Input: dimensioned drawing with shaded views. Units: mm. Origin: part minimum x, y, z. Round coordinates to 2 decimals unless told otherwise and drop trailing zeros. Order: outer loops, then holes, each group sorted by start corner. A loop starts at its lowest first (then second) coordinate and runs counter-clockwise, first axis right, second up. Notation, with made-up numbers: (85.25, -14.75) - (94.25, -14.75) arc R33 ccw to (94.25, 13.25) - close; hole circle Ø1 at (1, 44.25). An arc over 180 degrees is marked (long way). Put each result on its own line as item: value. Start each with the question number.
(1) Section D-D (x = 16.25). Output: boundary loops of the cut face in (y, z), and give its area (3 significant figures).
(2) Pin query (flat end, axial travel): P1, Ø1.5, axis at x = 5.5, z = 1, coming from the +Y side; P2, Ø1.6, axis at x = 4.5, y = 13.5, coming from the +Z side; P3, Ø1, axis at y = 14, z = 3.5, coming from the -X side; P4, Ø1.5, axis at x = 15, z = 1.5, coming from the +Y side. Return the tip coordinate at first contact, or that it passes through.
(3) Pull-direction query (X, two-part tool) for the marked faces 1, 2 and 3; classes: released by +X, released by -X, zero draft, split by the parting line, or undercut.
(4) Section B-B (x = 4.5). Output: boundary loops of the cut face in (y, z).
(5) Section A-A (z = 3.45). Output: boundary loops of the cut face in (x, y), and give its area (3 significant figures).
(6) Material intervals for L1, parallel to X at y = 4.5, z = 1.4; L2, parallel to Y at x = 4, z = 0.85, sorted ascending. Write a range as [from, to].
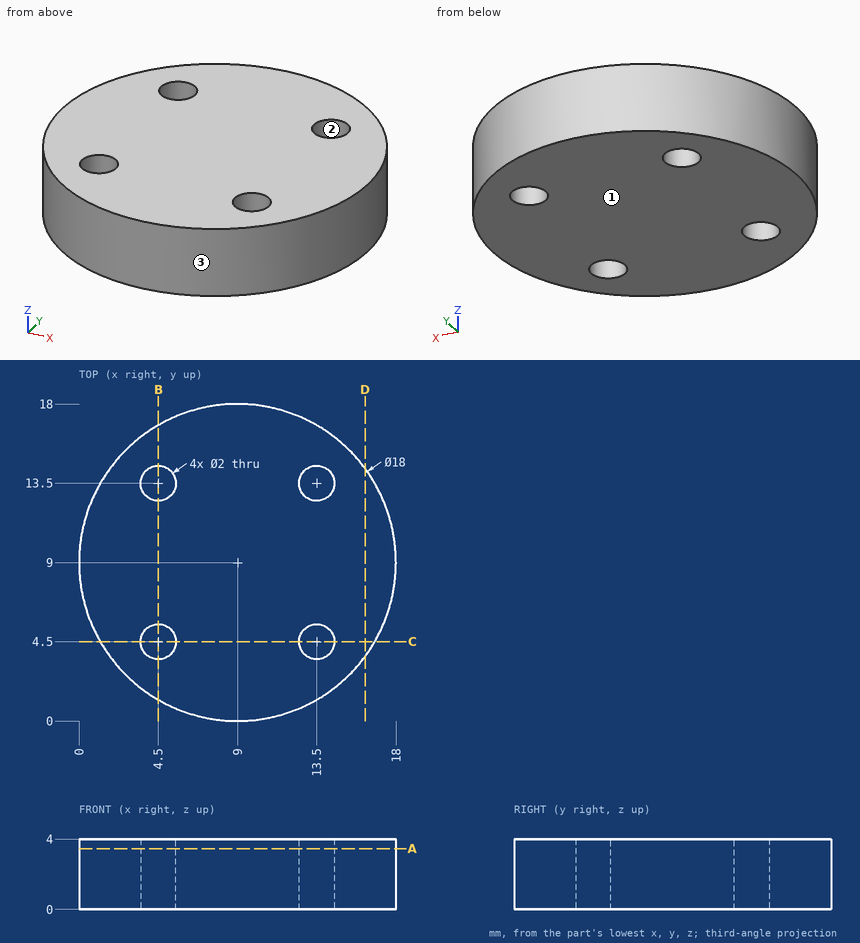
Checks:
1. outline: (3.67, 0) - (14.33, 0) - (14.33, 4) - (3.67, 4) - close
1. area: 42.7 mm²
2. P1: stops at y = 17.57
2. P2: passes through
2. P3: stops at x = 1.21
2. P4: stops at y = 16.31
3. face 1: zero draft
3. face 2: undercut
3. face 3: split by the parting line
4. outline: (1.21, 0) - (3.5, 0) - (3.5, 4) - (1.21, 4) - close; (5.5, 0) - (12.5, 0) - (12.5, 4) - (5.5, 4) - close; (14.5, 0) - (16.79, 0) - (16.79, 4) - (14.5, 4) - close
5. outline: circle Ø18 at (9, 9); hole circle Ø2 at (4.5, 4.5); hole circle Ø2 at (4.5, 13.5); hole circle Ø2 at (13.5, 4.5); hole circle Ø2 at (13.5, 13.5)
5. area: 242 mm²
6. L1: x = [1.21, 3.5], [5.5, 12.5], [14.5, 16.79]
6. L2: y = [1.52, 3.63], [5.37, 12.63], [14.37, 16.48]
